Work out the finished part from the listing and answer in its coordinate system (mm). A direction names the side the tool comes from. Round coordinates to 2 decimals unless told otherwise and drop trailing zeros. Order: outer loops, then holes, each group sorted by start corner. A loop starts at its lowest first (then second) coordinate and runs counter-clockwise, first axis right, second up. Notation, with made-up numbers: (41.25, 89) - (100.25, 89) arc R25 ccw to (100.25, 113) - close; hole circle Ø10 at (-18, 27). An arc over 180 degrees is marked (long way). Use one line per item in the form item = value. Start each with the question number.
Q1. Find the intervals of material crossed by line 1 (Y direction, x = 0, z = 10); line 2 (Z direction, x = 180.5, y = -121); line 3 (X direction, y = 0, z = -15), in increasing order. Write a range as [from, to].
Q2. The part is cut by section B-B on y = -117. State how many separate pieces and enclosed holes the cut face has, plus the area to 3 significant figures.
Q3. Which of the six approach directions +Z, -Z, +X, -X, +Y, -Y give full straight-line access (tool end or side, diameter ignored) to faces 1 (the cylindrical face through (23.61, 37.87, -30.07)), 2 (the flat face through (27, -40, 0)), 3 (the cylindrical face through (42.496, -0.565, 30.07))?
Q4. The part is cut by section A-A on z = -21. Determine the outline of the cut face in (x, y).
Q5. For a pull along X with two mould halves and no side action, classify faces 4 (the cylindrical face through (185, -117, -30)), 5 (the flat face through (153.47, -23.9, -0.45)), 6 (the cylindrical face through (218.899, -144.656, 29.972)), 7 (the flat face through (44, 40, 0)) as +X half, -X half, draft (parallel to the pull), parting line (faces both ways), or undercut.
Q6. Given P1, Ø1, axis at y = -39.5, z = 5, coming from the +X side; P2, Ø1, axis at y = -127.5, z = -13, coming from the -X side; P3, Ø11.5, axis at x = 190, y = -117, coming from the +Z side; P4, Ø1.5, axis at y = -101, z = 21.5, coming from the +X side, each flat-ended and moving along its own axis, determine where each tip first touches the part or whether it passes through.
Q7. The part is cut by section C-C on x = 37. Determine the outline of the cut face in (y, z), plus the area to 3 significant figures.
Autodesk Inventor part; units mm, degrees
ref_plane "YZ Plane" through (0, 0, 0) normal (1, 0, 0) x (0, 1, 0)
ref_plane "XZ Plane" through (0, 0, 0) normal (0, 1, 0) x (-1, 0, 0)
ref_plane "XY Plane" through (0, 0, 0) normal (0, 0, 1) x (1, 0, 0)
sketch "Sketch1" plane through (0, 0, 0) normal (0, 0, 1) x (1, 0, 0)
  arc A0 (0, 40) -> (0, -40) centre (0, 0) ccw
  arc A1 (161.7157, -145.2843) -> (218.2843, -88.7157) centre (190, -117) ccw
  line L0 (0, 40) -> (89.5685, 40)
  line L1 (89.5685, 40) -> (218.2843, -88.7157)
  line L2 (0, -40) -> (56.4315, -40)
  line L3 (56.4315, -40) -> (161.7157, -145.2843)
  arc A2 (0, -40) -> (0, 40) centre (0, 0) ccw construction
  arc A3 (218.2843, -88.7157) -> (161.7157, -145.2843) centre (190, -117) ccw construction
  circle A4 centre (0, 0) radius 5
  circle A5 centre (190, -117) radius 5
  line L4 (0, -40) -> (161.7157, -40)
  line L5 (93.4315, -77) -> (190, -77)
  dimension "d0" = 80
  dimension "d1" = 80
  dimension "d2" = 190
  dimension "d3" = 117
  dimension "d4" = 135
  dimension "d9" = 10
  dimension "d10" = 10
extrude "Extrusion1" add sketch "Sketch1" along normal mid plane 70
sketch "Sketch2" plane through (0, 0, 0) normal (0, 0, 1) x (1, 0, 0)
  arc A0 (0, 40) -> (0, -40) centre (0, 0) ccw
  line L0 (0, -40) -> (56.4315, -40)
  line L1 (56.4315, -40) -> (161.7157, -145.2843)
  arc A1 (161.7157, -145.2843) -> (218.2843, -88.7157) centre (190, -117) ccw
  line L2 (218.2843, -88.7157) -> (89.5685, 40)
  line L3 (89.5685, 40) -> (0, 40)
  circle A2 centre (0, 0) radius 42.5
  circle A3 centre (190, -117) radius 42.5
  point P0 (208.1292, -78.5607)
  point P1 (151.5607, -135.1292)
  dimension "d7" = 85
  dimension "d8" = 85
extrude "Extrusion2" cut sketch "Sketch2" along normal mid plane 50 contours L2 A1 L1 A3 picked at (179.9827, -106.9827)
sketch "Sketch3" plane through (0, 0, 35) normal (0, 0, 1) x (1, 0, 0)
  arc A0 (0, 40) -> (0, -40) centre (0, 0) ccw
  line L0 (0, -40) -> (56.4315, -40)
  line L1 (56.4315, -40) -> (161.7157, -145.2843)
  arc A1 (161.7157, -145.2843) -> (218.2843, -88.7157) centre (190, -117) ccw
  line L2 (218.2843, -88.7157) -> (89.5685, 40)
  line L3 (89.5685, 40) -> (0, 40)
  circle A2 centre (0, 0) radius 5
  circle A3 centre (190, -117) radius 5
  circle A4 centre (0, 0) radius 42.5
  dimension "d13" = 85
extrude "Extrusion3" cut sketch "Sketch3" against normal blind 10 contours L3 A4 L0 A0 | A0 L0 A4 L3 | A2
mirror "Mirror1" about plane through (0, 0, 0) normal (0, 0, 1) of "Extrusion3"
fillet "Fillet1" radius 3 24 edges at (14.3614, 40, -30) (14.3614, 40, 30) (14.3614, -40, 30) (14.3614, -40, -30) (151.5607, -135.1292, 0) (208.1292, -78.5607, 0) (51.965, 40, 35) (218.2843, -145.2843, 35) (109.0736, -92.6421, 35) (153.9264, -24.3579, 35) (51.965, 40, -35) (218.2843, -145.2843, -35) (109.0736, -92.6421, -35) (153.9264, -24.3579, -35) (89.5685, 40, 0) (56.4315, -40, 0) (35.3964, -40, 35) (35.3964, -40, -35) (213.2067, -83.6382, 25) (156.6382, -140.2067, 25) (218.2843, -145.2843, 25) (156.6382, -140.2067, -25) (213.2067, -83.6382, -25) (218.2843, -145.2843, -25)
properties part number "Arm2"
Found:
q1.line_1 = [-40, -5], [5, 40]
q1.line_2 = [-35, -25], [25, 35]
q1.line_3 = [-40, -5], [5, 129.57]
q2.separate_pieces = 3
q2.enclosed_holes = 0
q2.area = 2,420 mm²
q3.face_1 = -Z, -X
q3.face_2 = +Z, -Z, -X, -Y
q3.face_3 = +Z, -X
q4.outline = (0, -40) - (55.19, -40) arc R3 cw to (57.31, -40.88) - (142.99, -126.56) arc R3 ccw to (148.07, -123.95) arc R42.5 cw to (196.95, -75.07) arc R3 ccw to (199.56, -69.99) - (90.45, 39.12) arc R3 ccw to (88.33, 40) - (0, 40) arc R40 ccw to start; hole circle Ø10 at (0, 0)
q5.face_4 = undercut
q5.face_5 = +X half
q5.face_6 = parting line
q5.face_7 = draft
q6.P1 = 169.57
q6.P2 = 143.55
q6.P3 = 35
q6.P4 = 150.94
q7.outline = (-40, -32) arc R3 ccw to (-37, -35) - (-20.91, -35) - (-20.91, -25) - (20.91, -25) - (20.91, -35) - (37, -35) arc R3 ccw to (40, -32) - (40, 32) arc R3 ccw to (37, 35) - (20.91, 35) - (20.91, 25) - (-20.91, 25) - (-20.91, 35) - (-37, 35) arc R3 ccw to (-40, 32) - close
q7.area = 4,760 mm²
